Build history of the part. All positions in model axes, mm. Give positions to 0.01 mm unless a question says otherwise; leave off trailing zeros. Order: outer loops, then holes, each group sorted by start corner. A loop starts at its lowest first (then second) coordinate and runs counter-clockwise, first axis right, second up. Notation, with made-up numbers: M 88.5,85.5 L 144.5,85.5 A33 cw 144.5,114.5 Z; hole C 64,45 d6. An arc over 180 degrees is marked long. One line per item, written item: value.
from build123d import *

# Parameters (mm, degrees)
SKETCH1_W                = 23
SKETCH1_H                = 50
BASE_FLANGE1_DEPTH       = 1
SKETCH8_W                = 13
SKETCH8_H                = 24
CUT_EXTRUDE2_DEPTH       = 56.045435778
SKETCH9_W                = 17
SKETCH9_H                = 9
SKETCH9_W_2              = 3
SKETCH9_H_2              = 1
SKETCH9_H_3              = 25
SKETCH9_W_3              = 6
SKETCH9_H_4              = 2
CUT_EXTRUDE3_DEPTH       = 56.045435778
EDGE_FLANGE1_START       = -36.069185562
EDGE_FLANGE1_DEPTH       = 5.069185562
EDGE_FLANGE1_START_2     = -36.470498128
EDGE_FLANGE1_2_DEPTH     = 0.401312566
EDGE_FLANGE1_START_3     = 6
EDGE_FLANGE1_3_DEPTH     = 11
EDGE_FLANGE1_4_DEPTH     = 5.470498128
EDGE_FLANGE1_START_4     = -2.2366
EDGE_FLANGE1_5_OUTLINE_W = 0.5
EDGE_FLANGE1_5_OUTLINE_H = 1
EDGE_FLANGE1_5_DEPTH     = 0.2366
EDGE_FLANGE1_6_DEPTH     = 11
FILLET1_R                = 1
SKETCH19_W               = 4.427639712
SKETCH19_H               = 4
CUT_EXTRUDE4_DEPTH       = 48.528938553
SKETCH20_R               = 1
CUT_EXTRUDE5_DEPTH       = 48.528938553
SKETCH21_R               = 1
CUT_EXTRUDE6_DEPTH       = 10
CUT_EXTRUDE7_DEPTH       = 47.914816423
CUT_EXTRUDE7_DEPTH_BACK  = 10
SKETCH22_R               = 1
FILLET2_R                = 1


# Read off the part's stored shape, not the designer's step: Edge-Flange1
# Sheet-metal steps are written as plain solids
with BuildPart() as part:
    # Sketch1 → Base-Flange1 (new body)
    with BuildSketch(Plane(origin=(0, 0, 0), x_dir=(1, 0, 0), z_dir=(0, 1, 0))):
        with Locations((11.5, 25)):
            Rectangle(SKETCH1_W, SKETCH1_H)
    extrude(amount=-BASE_FLANGE1_DEPTH)

    # Sketch8 → Cut-Extrude2 (cut, through all)
    with BuildSketch(Plane.XZ.offset(1)):
        with Locations((11.5, -24.5)):
            Rectangle(SKETCH8_W, SKETCH8_H)
    extrude(amount=-CUT_EXTRUDE2_DEPTH, mode=Mode.SUBTRACT)

    # Sketch9 → Cut-Extrude3 (cut, through all)
    with BuildSketch(Plane.XZ.offset(1)):
        with Locations((11.5, -45.5)):
            Rectangle(SKETCH9_W, SKETCH9_H)
        Polygon((0, -50), (3, -50), (3, -41), (3, -36.470498128), (0, -36.470498128), align=None)
        Polygon((23, -50), (23, -36.069185562), (20, -36.069185562), (20, -41), (20, -50), align=None)
        with Locations((21.5, -30.5)):
            Rectangle(SKETCH9_W_2, SKETCH9_H_2)
        with Locations((1.5, -30.5)):
            Rectangle(SKETCH9_W_2, SKETCH9_H_2)
        with Locations((1.5, -14.5)):
            Rectangle(SKETCH9_W_2, SKETCH9_H_3)
        with Locations((20, -1)):
            Rectangle(SKETCH9_W_3, SKETCH9_H_4)
        with Locations((4.5, -1)):
            Rectangle(SKETCH9_W_2, SKETCH9_H_4)
        with Locations((1.5, -1)):
            Rectangle(SKETCH9_W_2, SKETCH9_H_4)
    extrude(amount=-CUT_EXTRUDE3_DEPTH, mode=Mode.SUBTRACT)

    # Edge-Flange1 outline → Edge-Flange1 (add)
    with BuildSketch(Plane.XY.offset(EDGE_FLANGE1_START)):
        with BuildLine():
            Line((23, 0.7366), (23, 6))
            Line((23, 6), (22, 6))
            Line((22, 6), (22, 0.7366))
            ThreePointArc((22, 0.7366), (21.784254855, 0.215745145), (21.2634, 0))
            Line((21.2634, 0), (22.83604109, 0))
            ThreePointArc((22.83604109, 0), (22.958514757, 0.359286442), (23, 0.7366))
        make_face()
        with BuildLine():
            Line((0.16395891, 0), (1.7366, 0))
            ThreePointArc((1.7366, 0), (1.215745145, 0.215745145), (1, 0.7366))
            Line((1, 0.7366), (1, 6))
            Line((1, 6), (0, 6))
            Line((0, 6), (0, 0.7366))
            ThreePointArc((0, 0.7366), (0.041485243, 0.359286442), (0.16395891, 0))
        make_face()
    extrude(amount=EDGE_FLANGE1_DEPTH)

    # Edge-Flange1 2 outline → Edge-Flange1 2 (add)
    with BuildSketch(Plane.XY.offset(EDGE_FLANGE1_START_2)):
        with BuildLine():
            Line((0.16395891, 0), (1.7366, 0))
            ThreePointArc((1.7366, 0), (1.215745145, 0.215745145), (1, 0.7366))
            Line((1, 0.7366), (1, 6))
            Line((1, 6), (0, 6))
            Line((0, 6), (0, 0.7366))
            ThreePointArc((0, 0.7366), (0.041485243, 0.359286442), (0.16395891, 0))
        make_face()
    extrude(amount=EDGE_FLANGE1_2_DEPTH)

    # Edge-Flange1 3 outline → Edge-Flange1 3 (add)
    with BuildSketch(Plane.YZ.offset(EDGE_FLANGE1_START_3)):
        with BuildLine():
            Line((6, 0), (0.7366, 0))
            ThreePointArc((0.7366, 0), (0.359286442, -0.041485243), (0, -0.16395891))
            Line((0, -0.16395891), (0, -1.7366))
            ThreePointArc((0, -1.7366), (0.215745145, -1.215745145), (0.7366, -1))
            Line((0.7366, -1), (6, -1))
            Line((6, -1), (6, 0))
        make_face()
    extrude(amount=EDGE_FLANGE1_3_DEPTH)

    # Edge-Flange1 4 outline → Edge-Flange1 4 (cut)
    with BuildSketch(Plane.XY.offset(EDGE_FLANGE1_START_2)):
        with BuildLine():
            Line((23, 0), (22.83604109, 0))
            ThreePointArc((22.83604109, 0), (22.195226164, -0.728828115), (21.2634, -1))
            Line((21.2634, -1), (23, -1))
            Line((23, -1), (23, 0))
        make_face()
        with BuildLine():
            Line((0, -1), (1.7366, -1))
            ThreePointArc((1.7366, -1), (0.804773836, -0.728828115), (0.16395891, 0))
            Line((0.16395891, 0), (0, 0))
            Line((0, 0), (0, -1))
        make_face()
    extrude(amount=EDGE_FLANGE1_4_DEPTH, mode=Mode.SUBTRACT)

    # Edge-Flange1 5 outline → Edge-Flange1 5 (cut)
    with BuildSketch(Plane.XY.offset(EDGE_FLANGE1_START_4)):
        with Locations((17.25, -0.5)):
            Rectangle(EDGE_FLANGE1_5_OUTLINE_W, EDGE_FLANGE1_5_OUTLINE_H)
        with Locations((5.75, -0.5)):
            Rectangle(EDGE_FLANGE1_5_OUTLINE_W, EDGE_FLANGE1_5_OUTLINE_H)
    extrude(amount=EDGE_FLANGE1_5_DEPTH, mode=Mode.SUBTRACT)

    # Edge-Flange1 6 outline → Edge-Flange1 6 (cut)
    with BuildSketch(Plane.YZ.offset(EDGE_FLANGE1_START_3)):
        with BuildLine():
            ThreePointArc((-1, -1.7366), (-0.728828115, -0.804773836), (0, -0.16395891))
            Line((0, -0.16395891), (0, 0))
            Line((0, 0), (-1, 0))
            Line((-1, 0), (-1, -1.7366))
        make_face()
    extrude(amount=EDGE_FLANGE1_6_DEPTH, mode=Mode.SUBTRACT)

    # Fillet1
    fillet1_edges = [part.edges().sort_by_distance(p)[0] for p in [
        (3, -0.5, -2),
        (0, -0.5, -27),
        (6, 6, -0.5),
        (17, 6, -0.5),
        (0.5, 6, -36.470498128),
        (0.5, 6, -31),
        (22.5, 6, -31),
        (22.5, 6, -36.069185562),
        (23, -0.5, -30),
        (0, -0.5, -30),
        (23, -0.5, -2),
    ]]
    fillet(fillet1_edges, radius=FILLET1_R)

    # Sketch19 → Cut-Extrude4 (cut, through all)
    with BuildSketch(Plane.XZ.offset(1)):
        with Locations((21.977182604, -13.849068818)):
            Rectangle(SKETCH19_W, SKETCH19_H)
    extrude(amount=-CUT_EXTRUDE4_DEPTH, mode=Mode.SUBTRACT)

    # Sketch20 → Cut-Extrude5 (cut, through all)
    with BuildSketch(Plane.XZ.offset(1)):
        with Locations(Location((7.5, -11, 0), (0, 0, 270))):
            Circle(SKETCH20_R)
        with Locations(Location((15.5, -11, 0), (0, 0, 270))):
            Circle(SKETCH20_R)
        with Locations(Location((7.5, -38, 0), (0, 0, 270))):
            Circle(SKETCH20_R)
        with Locations(Location((15.5, -38, 0), (0, 0, 270))):
            Circle(SKETCH20_R)
    extrude(amount=-CUT_EXTRUDE5_DEPTH, mode=Mode.SUBTRACT)

    # Sketch21 → Cut-Extrude6 (cut)
    with BuildSketch(Plane(origin=(0, 0, -1), x_dir=(-1, 0, 0), z_dir=(0, 0, -1))):
        with Locations((-11.5, 2.8683)):
            Circle(SKETCH21_R)
    extrude(amount=-CUT_EXTRUDE6_DEPTH, mode=Mode.SUBTRACT)

    # Sketch22 → Cut-Extrude7 (cut, two sides: drawn at the far end of the back side and taken through both)
    with BuildSketch(Plane.ZY.offset(-22).offset(-CUT_EXTRUDE7_DEPTH_BACK)):
        with Locations(Location((-33.534592781, 2.8683, 0), (0, 0, 90))):
            Circle(SKETCH22_R)
    extrude(amount=CUT_EXTRUDE7_DEPTH + CUT_EXTRUDE7_DEPTH_BACK, mode=Mode.SUBTRACT)

    # Fillet2
    fillet2_edges = [part.edges().sort_by_distance(p)[0] for p in [
        (3, -0.5, -41),
        (20, -0.5, -41),
    ]]
    fillet(fillet2_edges, radius=FILLET2_R)


solid = part.part
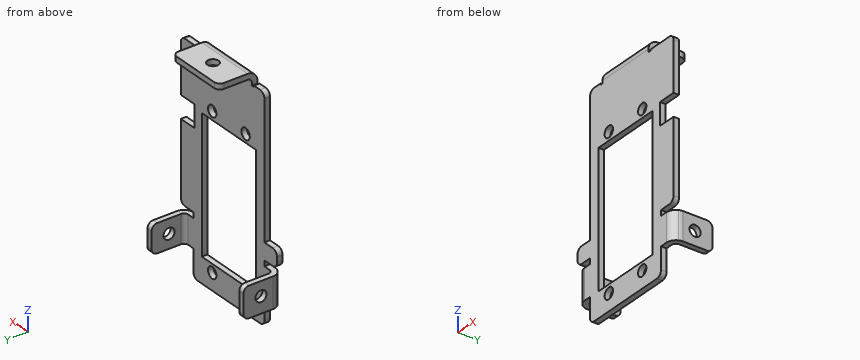
1) Saw through at B-B, the plane z = -22.5. Write the cut outline in (x, y), then the cut area to 3 significant figures.
Check values:
outline: M 3,-1 L 5,-1 L 5,0 L 3,0 Z; M 18,-1 L 23,-1 L 23,0 L 18,0 Z
area: 7.00 mm^2
2) Saw through at D-D, the plane z = -11. Write the cut outline in (x, y).
Check values:
outline: M 3,-1 L 6.5,-1 L 6.5,0 L 3,0 Z; M 8.5,-1 L 14.5,-1 L 14.5,0 L 8.5,0 Z; M 16.5,-1 L 23,-1 L 23,0 L 16.5,0 Z
3) Saw through at C-C, the plane x = 11.5. Write the cut outline in (y, z).
Check values:
outline: M -1,-41 L 0,-41 L 0,-36.5 L -1,-36.5 Z; M -1,-12.5 L 0,-12.5 L 0,-1.74 A0.74 cw 0.74,-1 L 1.87,-1 L 1.87,0 L 0.74,0 A1.74 ccw -1,-1.74 Z; M 3.87,-1 L 6,-1 L 6,0 L 3.87,0 Z
4) Drill centre lines: probe 1 along X at (y, z) = (-0.75, -11); probe 2 along X at (y, z) = (5.75, -33.5); probe 3 along X at (y, z) = (-0.5, -22). Where is each one in solid material? Low to high. Write a range as from..to.
Check values:
probe 1: 3..6.5, 8.5..14.5, 16.5..23
probe 2: 0..1, 22..23
probe 3: 3..5, 18..23
5) Pin check, flat tips, straight feed: pin 1 (1 mm diameter, centred on x = 18, z = -19, fed in from +Y); pin 2 (0.5 mm diameter, centred on y = -0.5, z = -37.5, fed in from +X); pin 3 (2.5 mm diameter, centred on x = 1.5, y = 1, fed in from +Z); pin 4 (4 mm diameter, centred on x = 13.5, y = 2.5, fed in from +Z). Stop position of each tip, or through.
Check values:
pin 1: y = 0
pin 2: x = 20
pin 3: z = -27
pin 4: z = 0
6) Saw through at A-A, the plane x = 15.5. Write the cut outline in (y, z), then the cut area to 3 significant figures.
Check values:
outline: M -1,-41 L 0,-41 L 0,-39 L -1,-39 Z; M -1,-37 L 0,-37 L 0,-36.5 L -1,-36.5 Z; M -1,-12.5 L 0,-12.5 L 0,-12 L -1,-12 Z; M -1,-10 L 0,-10 L 0,-1.74 A0.74 cw 0.74,-1 L 6,-1 L 6,0 L 0.74,0 A1.74 ccw -1,-1.74 Z
area: 18.5 mm^2
